The model under review builds one solid part; all positions refer to its coordinate system, in mm. A direction names the side the tool comes from. Give positions to 0.01 mm unless a question says otherwise; leave off trailing zeros. Loops run counter-clockwise (first coordinate to the right, second up) from the corner with the lowest first, then second, coordinate; pieces in that order, holes last. Notation, with made-up numbers: (42, -13) -> (85, -13) arc R26 cw to (85, 13) -> close; hole circle Ø4 at (79, -23). An arc over 180 degrees is marked (long way). Write each question's results on one line, items separated by ' | '. Start each with the question number.
Q1. Wall thickness on L1, parallel to Z at x = 0, y = 1; L2, parallel to Z at x = 0, y = 12; L3, parallel to X at y = 33.5, z = -9.5: over which ranges is each line inside the solid? List them lowest first. Write a range as [from, to].
Q2. Mouldability with a two-part tool opening along X and no side actions: class faces 4 (the face through (-24, 60, -8)), 5 (the face through (-23.846, 29.58, -7.509)), 6 (the face through (5.85, 29.58, 26.36)) as released by +X, released by -X, zero draft, split by the parting line, or undercut.
Q3. We need section A-A (z = -6). Write out the cut boundary in (x, y).
Q4. We need section B-B (z = -15). Write out the cut boundary in (x, y).
Q5. We need section C-C (y = 25). Write out the cut boundary in (x, z).
Q6. Insertion check: pin 1 Ø1 at (y, z) = (37.5, 12) entering from -X; pin 2 Ø6 at (y, z) = (42, 3.5) entering from -X; pin 3 Ø5 at (x, z) = (1, 3.5) entering from +Y; pin 4 Ø2.5 at (x, z) = (-5.66, -5.66) entering from -Y. Each pin has a flat end and moves straight along its axis. Give the tip position at first contact, or say it passes through.
Q7. We need section D-D (z = 17). Write out the cut boundary in (x, y).
Q8. Machinability: for faces 1 (the face through (0, 0, -2)), 2 (the face through (7.99, 0.99, -10.82)), 3 (the face through (-0.1, 2, -2.7)), which of the approach directions +Z, -Z, +X, -X, +Y, -Y give a long, thin tool a straight path to every point of the face, cutting with its end or side? Answer none if there is none.
Autodesk Inventor part; units mm, degrees
ref_plane "YZ Plane" through (0, 0, 0) normal (1, 0, 0) x (0, 1, 0)
ref_plane "XZ Plane" through (0, 0, 0) normal (0, 1, 0) x (-1, 0, 0)
ref_plane "XY Plane" through (0, 0, 0) normal (0, 0, 1) x (1, 0, 0)
sketch "草圖1" plane through (0, 0, 0) normal (0, 1, 0) x (-1, 0, 0)
  circle A0 centre (0, 0) radius 25
  circle A1 centre (0, 0) radius 27
  dimension "d0" = 50
  dimension "d1" = 2
extrude "擠出1" add sketch "草圖1" along normal blind 60
sketch "草圖2" plane through (0, 0, 0) normal (0, -1, 0) x (1, 0, 0)
  circle A0 centre (0, 0) radius 25 construction
  line L0 (-25, 0) -> (25, 0) construction
  line L1 (-17.6777, 17.6777) -> (17.6777, -17.6777) construction
  line L2 (-16.2068, 19.0352) -> (19.0352, -16.2068)
  line L3 (-19.0352, 16.2068) -> (16.2068, -19.0352)
  arc A1 (-16.2068, 19.0352) -> (-19.0352, 16.2068) centre (0, 0) ccw
  arc A2 (16.2068, -19.0352) -> (19.0352, -16.2068) centre (0, 0) ccw
  line L4 (-19.0352, -16.2068) -> (16.2068, 19.0352)
  arc A3 (-19.0352, -16.2068) -> (-16.2068, -19.0352) centre (0, 0) ccw
  line L5 (-16.2068, -19.0352) -> (19.0352, 16.2068)
  arc A4 (19.0352, 16.2068) -> (16.2068, 19.0352) centre (0, 0) ccw
  dimension "d10" = 45
  dimension "d11" = 2
  dimension "d14" = 90
extrude "擠出3" add sketch "草圖2" against normal blind 2
sketch "草圖5" plane through (0, 0, 0) normal (0, -1, 0) x (1, 0, 0)
  circle A0 centre (0, 0) radius 25 construction
  line L0 (17.6777, 17.6777) -> (-17.6777, -17.6777) construction
  line L1 (-17.6777, 17.6777) -> (17.6777, -17.6777) construction
  line L2 (-25, 0) -> (25, 0) construction
  arc A1 (19.0352, -16.2068) -> (19.0352, 16.2068) centre (0, 0) ccw construction
  point P0 (5.6569, 5.6569)
  point P1 (-6.7175, 6.7175)
  point P2 (0, 0)
  point P3 (-5.6569, -5.6569)
  point P4 (6.7175, -6.7175)
  dimension "d18" = 45
  dimension "d19" = 45
  dimension "d20" = 9.5
  dimension "d21" = 8
  dimension "d24" = 180
hole "孔1" at (0, 0, 0) at (5.6569, 0, 5.6569) at (-6.7175, 0, 6.7175) at (-5.6569, 0, -5.6569) at (6.7175, 0, -6.7175) direction (0, 1, 0) diameter 3 end through all
Output:
1) L1: [-27, -25], [-2.83, -1.5], [1.5, 2.83], [25, 27] | L2: [-27, -25], [25, 27] | L3: [-25.27, -23.12], [23.12, 25.27]
2) face 4: zero draft | face 5: undercut | face 6: split by the parting line
3) outline: (-26.32, 0) -> (-24.27, 0) -> (-24.27, 60) -> (-26.32, 60) -> close; (-8.83, 0) -> (-7.12, 0) -> (-7.12, 2) -> (-8.83, 2) -> close; (-4.2, 0) -> (-3.17, 0) -> (-3.17, 2) -> (-4.2, 2) -> close; (3.17, 0) -> (5.4, 0) -> (5.4, 2) -> (3.17, 2) -> close; (8.03, 0) -> (8.83, 0) -> (8.83, 2) -> (8.03, 2) -> close; (24.27, 0) -> (26.32, 0) -> (26.32, 60) -> (24.27, 60) -> close
4) outline: (-22.45, 0) -> (-20, 0) -> (-20, 60) -> (-22.45, 60) -> close; (-17.83, 0) -> (-12.17, 0) -> (-12.17, 2) -> (-17.83, 2) -> close; (12.17, 0) -> (17.83, 0) -> (17.83, 2) -> (12.17, 2) -> close; (20, 0) -> (22.45, 0) -> (22.45, 60) -> (20, 60) -> close
5) outline: circle Ø54 at (0, 0); hole circle Ø50 at (0, 0)
6) pin 1: x = -24.43 | pin 2: x = -27 | pin 3: y = 2 | pin 4: through
7) outline: (-20.98, 0) -> (-14.17, 0) -> (-14.17, 2) -> (-18.33, 2) -> (-18.33, 60) -> (-20.98, 60) -> close; (14.17, 0) -> (20.98, 0) -> (20.98, 60) -> (18.33, 60) -> (18.33, 2) -> (14.17, 2) -> close
8) face 1: +Z, -Z, +X, -X, -Y | face 2: +Y, -Y | face 3: +Y
